Could you check a few things on this model? Use its own coordinates, in mm. A direction names the side the tool comes from. Coordinates: 2 decimals unless noted, no trailing zeros. Order: outer loops, then holes, each group sorted by start corner. A loop starts at its lowest first (then second) coordinate and runs counter-clockwise, first axis right, second up. Notation, with made-up numbers: (-39, -19.5) -> (-30, -19.5) arc R12 cw to (-30, 2.5) -> close; hole circle Ø5 at (78.25, 74). An arc over 180 degrees is marked (long way). Put each result on its own line as item: value. Start each with the question number.
Q1. For faces 1 (the face through (-0.13, -10.978, 13.037)), 2 (the face through (-9.5, -1.1, 11.206)), which set-ups out of +Z, -Z, +X, -X, +Y, -Y let a thin tool reach every point of the face, with its end or its side?
Q2. If we section it at A-A (z = 15.2): Please give me the cut outline in (x, y).
Q3. Will these pins go through, and if not, where does the flat tip stop? pin 1 (2.5 mm diameter, centred on x = -1, y = -0.5, fed in from -Z); pin 2 (2 mm diameter, centred on y = 1, z = 13.5, fed in from +X); pin 3 (1.5 mm diameter, centred on x = -1.5, z = 15, fed in from +Y).
Q4. We'd pull the mould along Y, two halves only. Please class faces 3 (the face through (-7.83, -0.2, 14.1)), 4 (the face through (0.13, 10.911, 13.104)), 5 (the face through (-0.12, -12.01, 13.42)): +Y half, -Y half, draft (parallel to the pull), parting line (faces both ways), or undercut.
Q5. If we section it at C-C (z = 13.75): Please give me the cut outline in (x, y).
Q6. If we section it at D-D (x = -7.5): Please give me the cut outline in (y, z).
Q7. Please list where these lines run through material, in increasing order: line 1 along Y through (x, z) = (-4, 11.65); line 2 along Z through (x, y) = (0.5, -7.5); line 3 along Y through (x, z) = (-1, 15.7).
Q8. If we section it at B-B (x = -2.25): Please give me the cut outline in (y, z), and give its area (3 significant figures).
from build123d import *

# Parameters (mm, degrees)
F0_W      = 16.1028504372
F0_H      = 24.0115216002
F2_W      = 24
F2_H      = 31
F5_W      = 14.02631565
F5_H      = 35.0832007825
F6_DEPTH  = 5
F8_W      = 36.7084983736
F8_H      = 15.6723505352
F9_DEPTH  = 5
F11_W     = 29.3105235323
F11_H     = 18.8404771034
F12_DEPTH = 5
F14_W     = 31.5226018429
F14_H     = 13.2806529291
F15_DEPTH = 5
F16_W     = 23.4492318705
F16_H     = 12.546513346
F17_DEPTH = 25.4
F18_T     = 1


# Not quite as in the source:
# - a shell that OpenCascade refuses in one call is made with other operations: the cavity is built on its own and cut out


with BuildPart() as f3:
    # F0 (on Top) → F3 section 0
    with BuildSketch(Plane.XY):
        with Locations((0.0935448334, 0.0057467259)):
            Rectangle(F0_W, F0_H)
    # F2 (on offset) → F3 section 1
    with BuildSketch(Plane.XY.offset(17)):
        Rectangle(F2_W, F2_H)
    loft()

    # F5 (on face) → F6 (cut)
    with BuildSketch(Plane(origin=(-14.5, 0, 14.5), x_dir=(0.7071067812, 0, 0.7071067812), z_dir=(0.7071067812, 0, -0.7071067812))):
        with Locations((2.1269769641, -0.2655759454)):
            Rectangle(F5_W, F5_H)
    extrude(amount=F6_DEPTH, mode=Mode.SUBTRACT)

    # F8 (on face) → F9 (cut)
    with BuildSketch(Plane(origin=(14.5, 0, 14.5), x_dir=(0, 1, 0), z_dir=(0.7071067812, 0, 0.7071067812))):
        with Locations((-0.0566011295, 4.1208126349)):
            Rectangle(F8_W, F8_H)
    extrude(amount=-F9_DEPTH, mode=Mode.SUBTRACT)

    # F11 (on face) → F12 (cut)
    with BuildSketch(Plane(origin=(0, 16.25, 16.25), x_dir=(-1, 0, 0), z_dir=(0, 0.7071067812, 0.7071067812))):
        with Locations((0.3414950334, 3.7744397996)):
            Rectangle(F11_W, F11_H)
    extrude(amount=-F12_DEPTH, mode=Mode.SUBTRACT)

    # F14 (on face) → F15 (cut)
    with BuildSketch(Plane(origin=(0, -16.25, 16.25), x_dir=(1, 0, 0), z_dir=(0, 0.7071067812, -0.7071067812))):
        with Locations((0.8808970451, -0.6048630457)):
            Rectangle(F14_W, F14_H)
    extrude(amount=F15_DEPTH, mode=Mode.SUBTRACT)

    # F16 (on Front) → F17 (cut, symmetric)
    with BuildSketch(Plane.XZ):
        with Locations((-0.0993120484, 4.9331299379)):
            Rectangle(F16_W, F16_H)
    extrude(amount=F17_DEPTH, both=True, mode=Mode.SUBTRACT)

    # F18: shell of thickness 1, made by hand


with BuildPart() as f18_core1:
    # F18_t2: copy of F3
    add(f3.part)

    # the walls: a layer under each face that stays
    f18_faces = [f18_core1.faces().sort_by_distance(p)[0] for p in [
        (10.6895617231, -5.424e-06, 11.2211990551),
        (0.0256243836, -11.3257388827, 14.1031933054),
        (7.8109264385, 0, 14.1180057497),
        (0.0256243836, 11.3257388827, 14.1031933054),
        (0, 0, 17),
        (-7.7853020549, 0, 14.1436301332),
        (-10.6320571867, -1.4807e-05, 11.2468234387),
    ]]
    thicken(f18_faces, amount=-F18_T, mode=Mode.SUBTRACT)


with BuildPart() as f3_1:
    add(f3.part)

    # what is left inside the walls is the cavity
    f18_cavity = [f18_core1.part.solids().sort_by_distance(p)[0] for p in [
        (0, 4.269444, 11.216387),
    ]]
    add(f18_cavity, mode=Mode.SUBTRACT)


solid = f3_1.part
The answers:
1. face 1: -Z
1. face 2: -Z, +X, -X, +Y, -Y
2. outline: (-6.73, -10.23) -> (6.73, -10.23) -> (6.73, 10.23) -> (-6.73, 10.23) -> close; hole (-5.31, -8.81) -> (5.31, -8.81) -> (5.31, 8.81) -> (-5.31, 8.81) -> close
3. pin 1: z = 16
3. pin 2: x = 9.43
3. pin 3: y = 11.18
4. face 3: draft
4. face 4: undercut
4. face 5: -Y half
5. outline: (-8.18, -11.68) -> (8.18, -11.68) -> (8.18, 11.68) -> (-8.18, 11.68) -> close; hole (-6.76, -10.26) -> (6.76, -10.26) -> (6.76, 10.26) -> (-6.76, 10.26) -> close
6. outline: (-14.22, 11.21) -> (-12.81, 11.21) -> (-11, 13.01) -> (11, 13.01) -> (12.81, 11.21) -> (14.22, 11.21) -> (11, 14.43) -> (-11, 14.43) -> close
7. line 1: -13.78 to -12.36, 12.36 to 13.78
7. line 2: 16 to 17
7. line 3: -9.73 to -8.31, 8.31 to 9.73
8. outline: (-14.22, 11.21) -> (-12.81, 11.21) -> (-8.01, 16) -> (8.01, 16) -> (12.81, 11.21) -> (14.22, 11.21) -> (8.43, 17) -> (-8.43, 17) -> close
8. area: 31.4 mm^2
